Can you work these out from the drawing? Everything is in mm from the part's minimum corner. A direction names the side the tool comes from. Coordinates: 2 decimals unless noted, no trailing zeros. Loops run counter-clockwise (first coordinate to the right, second up) from the corner with the lowest first, then second, coordinate; pieces in that order, holes last.
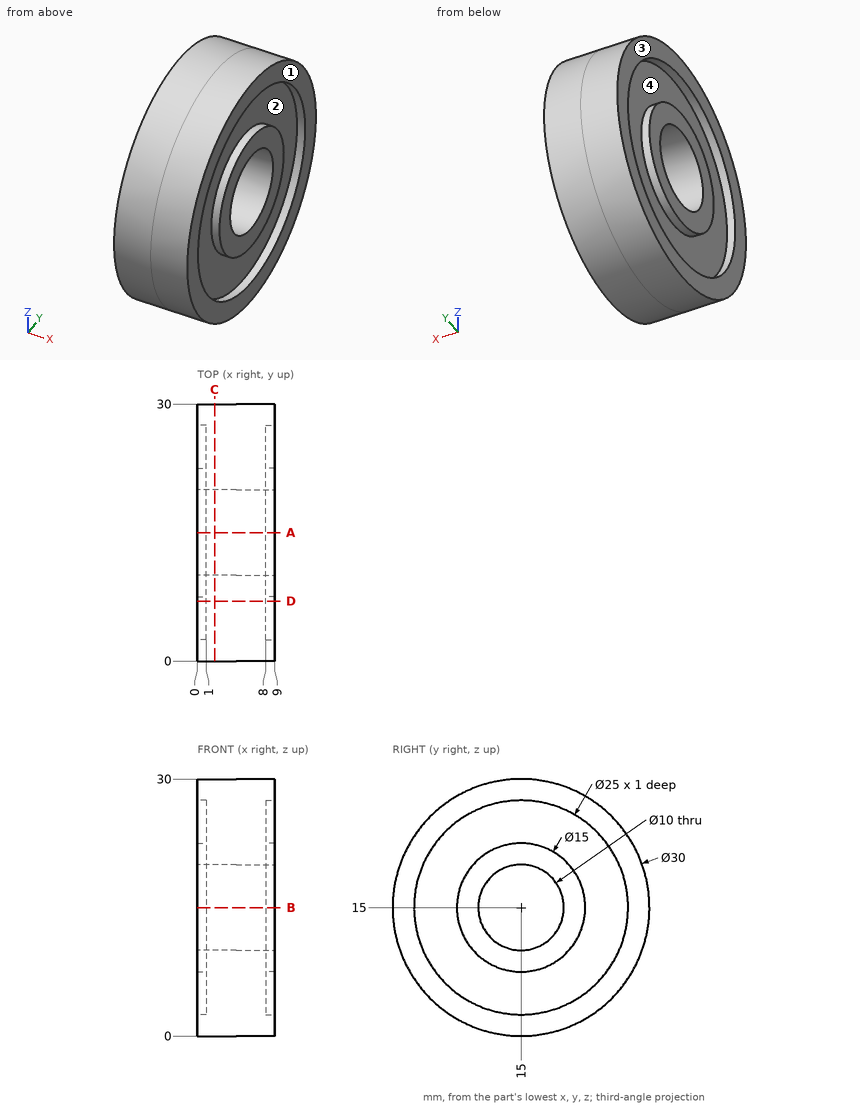
Item 1: I'm going to push flat-ended pins straight in: P1, Ø1.5, axis at x = 6, z = 3, coming from the -Y side; P2, Ø5, axis at x = 1.5, y = 18.5, coming from the +Z side; P3, Ø9, axis at y = 15, z = 15, coming from the -X side. Where does each tip first touch, or does it pass through?
Results are:
P1: stops at y = 5.08
P2: stops at z = 29.97
P3: passes through
Item 2: We'd pull the mould along Y, two halves only. Please class the marked faces 3 and 4: +Y half, -Y half, draft (parallel to the pull), parting line (faces both ways), or undercut.
Results are:
face 3: draft
face 4: undercut
Item 3: On a 3-axis mill with a long thin cutter (end or side, diameter ignored), from which of +Z, -Z, +X, -X, +Y, -Y can I reach the whole of each face in a straight line? I mean the marked faces 1 and 2. Say none if no direction works.
Results are:
face 1: +Z, -Z, +X, +Y, -Y
face 2: +X
Item 4: Suppose I cut it at D-D, the plane y = 7. Please give me the cut outline in (x, z).
Results are:
outline: (0, 2.31) - (9, 2.31) - (9, 5.4) - (8, 5.4) - (8, 24.6) - (9, 24.6) - (9, 27.69) - (0, 27.69) - (0, 24.6) - (1, 24.6) - (1, 5.4) - (0, 5.4) - close
Item 5: Suppose I cut it at A-A, the plane y = 15. Please give me the cut outline in (x, z), plus the area to 3 significant figures.
Results are:
outline: (0, 0) - (9, 0) - (9, 2.5) - (8, 2.5) - (8, 7.5) - (9, 7.5) - (9, 10) - (0, 10) - (0, 7.5) - (1, 7.5) - (1, 2.5) - (0, 2.5) - close; (0, 20) - (9, 20) - (9, 22.5) - (8, 22.5) - (8, 27.5) - (9, 27.5) - (9, 30) - (0, 30) - (0, 27.5) - (1, 27.5) - (1, 22.5) - (0, 22.5) - close
area: 160 mm2
Item 6: Suppose I cut it at C-C, the plane x = 2. Please give me the cut outline in (y, z), plus the area to 3 significant figures.
Results are:
outline: circle Ø30 at (15, 15); hole circle Ø10 at (15, 15)
area: 628 mm2
Item 7: I need wall thicknesses on line 1 along Y through (x, z) = (0.5, 15); line 2 along Y through (x, z) = (6.75, 15); line 3 along Z through (x, y) = (5, 14.75). Which ranges of each line are inside material? Lowest first, please.
Results are:
line 1: y = 0 to 2.5, 7.5 to 10, 20 to 22.5, 27.5 to 30
line 2: y = 0 to 10, 20 to 30
line 3: z = 0 to 10.01, 19.99 to 30
